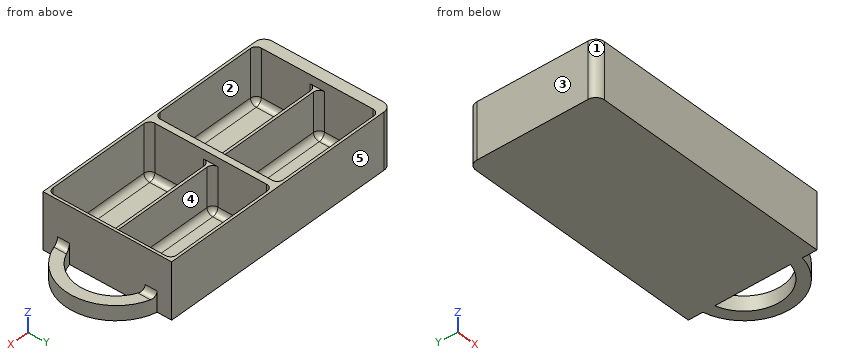
```python
from build123d import *

# Parameters (mm, degrees)
SKETCH_1_W                  = 86
SKETCH_1_H                  = 44.2
EXTRUDE_1_DEPTH             = 14.2
EXTRUDE_2_DEPTH             = 5
SKETCH_3_W                  = 81.1
SKETCH_3_H                  = 42.4
CUT_EXTRUDE_1_DEPTH         = 18.3
HOLE_WIZARD_8_3_8_3_1_D     = 8.3
HOLE_WIZARD_8_3_8_3_1_DEPTH = 3.2
RIB_1_REACH                 = 108.755
SKETCH_6_WALL_W             = 296.60943773
SKETCH_6_WALL_H             = 0.9
FILLET_1_R                  = 3
EXTRUDE_START               = -3.5
SKETCH_7_R                  = 4.15
EXTRUDE_3_DEPTH             = 3.5
FILLET_2_R                  = 2
SKETCH_9_W                  = 2.2
SKETCH_9_H                  = 19.2
EXTRUDE_4_DEPTH             = 44
FILLET_3_R                  = 2


with BuildPart() as part:
    # Эскиз1 → Бобышка-Вытянуть1 (new body)
    with BuildSketch(Plane.XY.offset(9.6)):
        with Locations((47, 0)):
            Rectangle(SKETCH_1_W, SKETCH_1_H)
    extrude(amount=-EXTRUDE_1_DEPTH)

    # Эскиз2 → Бобышка-Вытянуть2 (add)
    with BuildSketch(Plane(origin=(0, 0, -4.6), x_dir=(-1, 0, 0), z_dir=(0, 0, -1))):
        with BuildLine():
            Line((-90, -22.1), (-90, -17.1))
            ThreePointArc((-90, -17.1), (-104, 0), (-90, 17.1))
            Line((-90, 17.1), (-90, 22.1))
            Line((-90, 22.1), (-4, 22.1))
            Line((-4, 22.1), (-4, -22.1))
            Line((-4, -22.1), (-90, -22.1))
        make_face()
        with BuildLine():
            Line((-90, -12.994779171), (-90, 12.994779171))
            ThreePointArc((-90, 12.994779171), (-100, 0), (-90, -12.994779171))
        make_face(mode=Mode.SUBTRACT)
    extrude(amount=EXTRUDE_2_DEPTH)

    # Эскиз3 → Вырез-Вытянуть1 (cut)
    with BuildSketch(Plane.XY.offset(9.6)):
        with Locations((48.55, 0)):
            Rectangle(SKETCH_3_W, SKETCH_3_H)
    extrude(amount=-CUT_EXTRUDE_1_DEPTH, mode=Mode.SUBTRACT)

    # Диаметр отверстия Ø8.3 (8.3)1
    with Locations(Plane.ZY.offset(-4)):
        with Locations((0, 0)):
            Hole(HOLE_WIZARD_8_3_8_3_1_D / 2, depth=HOLE_WIZARD_8_3_8_3_1_DEPTH)

    # Эскиз6 wall → Ребро1 (add, up to next)
    with BuildSketch(Plane(origin=(48.55, 0, 6.6), x_dir=(1, 0, 0), z_dir=(0, 0, -1)), mode=Mode.PRIVATE) as rib_1_sk1:
        Rectangle(SKETCH_6_WALL_W, SKETCH_6_WALL_H)
    rib_1_tool1 = extrude(rib_1_sk1.sketch, amount=RIB_1_REACH, mode=Mode.PRIVATE) - part.part
    add(rib_1_tool1.solids().sort_by_distance((48.55, 0, 6.6))[0])

    # Скругление1
    fillet_1_edges = [part.edges().sort_by_distance(p)[0] for p in [
        (4, -22.1, 0),
        (4, 22.1, 0),
    ]]
    fillet(fillet_1_edges, radius=FILLET_1_R)

    # Эскиз7 → Бобышка-Вытянуть3 (add)
    with BuildSketch(Plane.ZY.offset(-4).offset(EXTRUDE_START)):
        Circle(SKETCH_7_R)
    extrude(amount=EXTRUDE_3_DEPTH)

    # Скругление2
    fillet_2_edges = [part.edges().sort_by_distance(p)[0] for p in [
        (90, -15.047389586, -4.6),
        (90, 15.047389586, -4.6),
        (8, 10.825, -8.7),
        (8, -21.2, 0.45),
        (48.55, 21.2, -8.7),
        (8, 21.2, 0.45),
        (89.1, -10.825, -8.7),
        (89.1, 21.2, 0.45),
        (48.55, -21.2, -8.7),
        (89.1, -21.2, 0.45),
        (8, -10.825, -8.7),
        (89.1, 10.825, -8.7),
        (48.55, 0.45, -8.7),
        (8, 0.45, -1.05),
        (89.1, 0.45, -1.05),
        (8, -0.45, -1.05),
        (89.1, -0.45, -1.05),
        (48.55, -0.45, -8.7),
    ]]
    fillet(fillet_2_edges, radius=FILLET_2_R)

    # Эскиз9 → Бобышка-Вытянуть4 (add)
    with BuildSketch(Plane(origin=(0, 22.1, 0), x_dir=(1, 0, 0), z_dir=(0, 1, 0))):
        with Locations((48.5, 0)):
            Rectangle(SKETCH_9_W, SKETCH_9_H)
    extrude(amount=-EXTRUDE_4_DEPTH)

    # Скругление3
    fillet_3_edges = [part.edges().sort_by_distance(p)[0] for p in [
        (47.4, 1.035786438, -8.114213562),
        (49.6, 1.035786438, -8.114213562),
        (49.6, -10.825, -8.7),
        (49.6, 0.45, -0.05),
        (49.6, 10.825, -8.7),
        (47.4, 10.825, -8.7),
        (47.4, 0.45, -0.05),
        (47.4, -10.825, -8.7),
        (49.6, -20.614213562, -8.114213562),
        (49.6, -21.2, 1.45),
        (49.6, 21.2, 1.45),
        (49.6, 20.614213562, -8.114213562),
        (49.6, -0.45, -0.05),
        (49.6, -1.035786438, -8.114213562),
        (47.4, -21.2, 1.45),
        (47.4, -20.614213562, -8.114213562),
        (47.4, -1.035786438, -8.114213562),
        (47.4, -0.45, -0.05),
        (47.4, 20.614213562, -8.114213562),
        (47.4, 21.2, 1.45),
    ]]
    fillet(fillet_3_edges, radius=FILLET_3_R)


solid = part.part
```
Model file for the job. Use its own axes, mm. Face numbers are marked on the shaded views. A direction names the side the tool comes from. Round coordinates to 2 decimals unless told otherwise and drop trailing zeros. Write each loop counter-clockwise with the first axis right and the second up, starting at its lowest first coordinate (ties: lowest second). Pieces come first, ordered by that corner, then holes. Notation, with made-up numbers: M -9.75,-12 L 40.25,-12 A20 cw 40.25,15 Z; hole C 19.25,5 d4. An arc over 180 degrees is marked long. Put each result on its own line as item: value.
Item 1: Tool access for the marked faces 1 and 2: list every direction of +Z, -Z, +X, -X, +Y, -Y with a clear straight run to the whole face (end or side of a thin tool).
Responses:
face 1: +Z, -Z, -X, -Y
face 2: +Z
Item 2: Cut at C-C (x = 36). List the corners of the cut face in (y, z).
Responses:
outline: M -22.1,-9.6 L 22.1,-9.6 L 22.1,9.6 L 21.2,9.6 L 21.2,-6.7 A2 cw 19.2,-8.7 L 2.45,-8.7 A2 cw 0.45,-6.7 L 0.45,6.6 L -0.45,6.6 L -0.45,-6.7 A2 cw -2.45,-8.7 L -19.2,-8.7 A2 cw -21.2,-6.7 L -21.2,9.6 L -22.1,9.6 Z
Item 3: Cut at A-A (z = 8). List the corners of the cut face in (x, y), and give its area (3 significant figures).
Responses:
outline: M 4,-19.1 A3 ccw 7,-22.1 L 90,-22.1 L 90,22.1 L 7,22.1 A3 ccw 4,19.1 Z; hole M 8,-19.2 A2 ccw 10,-21.2 L 45.4,-21.2 A2 ccw 47.4,-19.2 L 47.4,19.2 A2 ccw 45.4,21.2 L 10,21.2 A2 ccw 8,19.2 Z; hole M 49.6,-19.2 A2 ccw 51.6,-21.2 L 87.1,-21.2 A2 ccw 89.1,-19.2 L 89.1,19.2 A2 ccw 87.1,21.2 L 51.6,21.2 A2 ccw 49.6,19.2 Z
area: 459 mm²
Item 4: Cut at D-D (z = 2). State how many separate pieces and enclosed holes the cut face has, and give its area (3 significant figures).
Responses:
separate pieces: 1
enclosed holes: 4
area: 537 mm²
Item 5: Cut at B-B (y = -10.5). List the corners of the cut face in (x, z).
Responses:
outline: M 4,-9.6 L 90,-9.6 L 90,9.6 L 89.1,9.6 L 89.1,-6.7 A2 cw 87.1,-8.7 L 51.6,-8.7 A2 cw 49.6,-6.7 L 49.6,9.6 L 47.4,9.6 L 47.4,-6.7 A2 cw 45.4,-8.7 L 10,-8.7 A2 cw 8,-6.7 L 8,9.6 L 4,9.6 Z; M 94.95,-9.6 L 100.49,-9.6 L 100.49,-4.6 L 94.95,-4.6 Z
Item 6: Flat gauge pins, fed straight in: P1, Ø4, axis at x = 52, y = 3.5, coming from the +Z side; P2, Ø1.5, axis at y = -13.5, z = -7, coming from the +X side; P3, Ø5.5, axis at x = 36.5, y = 1, coming from the +Z side. Where does each tip first touch, or does it go through?
Responses:
P1: z = -7.9
P2: x = 98.46
P3: z = 6.6
Item 7: Mould opens along X. For the marked faces 3, 4 and 5 say: +X half, -X half, draft (parallel to the pull), parting line (faces both ways), or undercut.
Responses:
face 3: -X half
face 4: undercut
face 5: draft
Item 8: Probe L1, parallel to X at y = 10.5, z = -3.5; L2, parallel to Y at x = 15.5, z = 3; L3, parallel to Y at x = 45.5, z = 7.5. List the from-to ranges inside material, lowest first. Write a range as from..to.
Responses:
L1: 4..8, 47.4..49.6, 89.1..90
L2: -22.1..-21.2, -0.45..0.45, 21.2..22.1
L3: -22.1..-21.2, 21.2..22.1
